Source: CAD feature listing. Evaluate the final solid. Frame: model axes, mm. A direction names the side the tool comes from. Give positions to 0.01 mm unless a question says otherwise; leave off trailing zeros. Order: outer loops, then holes, each group sorted by start corner. A loop starts at its lowest first (then second) coordinate and runs counter-clockwise, first axis right, second up.
from build123d import *

# Parameters (mm, degrees)
SKETCH1_W           = 500
SKETCH1_H           = 150
BOSS_EXTRUDE1_DEPTH = 10
SKETCH2_R           = 25.831615562
CUT_EXTRUDE1_DEPTH  = 10
SKETCH3_W           = 401.190926376
SKETCH3_H           = 128.182737921
CUT_EXTRUDE2_DEPTH  = 10
SKETCH5_W           = 641.31413219
SKETCH5_H           = 43.634524158
CUT_EXTRUDE3_DEPTH  = 10


with BuildPart() as part:
    # Sketch1 → Boss-Extrude1 (new body)
    with BuildSketch(Plane.XY):
        Rectangle(SKETCH1_W, SKETCH1_H)
    extrude(amount=BOSS_EXTRUDE1_DEPTH)

    # Sketch2 → Cut-Extrude1 (cut)
    with BuildSketch(Plane.XY.offset(10)):
        with Locations((195.256623511, 25)):
            Circle(SKETCH2_R)
    extrude(amount=-CUT_EXTRUDE1_DEPTH, mode=Mode.SUBTRACT)

    # Sketch3 → Cut-Extrude2 (cut)
    with BuildSketch(Plane.XY.offset(10)):
        with Locations((-49.404536812, 10.908631039)):
            Rectangle(SKETCH3_W, SKETCH3_H)
    extrude(amount=-CUT_EXTRUDE2_DEPTH, mode=Mode.SUBTRACT)

    # Sketch5 → Cut-Extrude3 (cut)
    with BuildSketch(Plane.XY.offset(10)):
        with Locations((-250, -53.182737921)):
            Rectangle(SKETCH5_W, SKETCH5_H)
    extrude(amount=-CUT_EXTRUDE3_DEPTH, mode=Mode.SUBTRACT)


solid = part.part
(1) Access query for faces 4 (the flat face through (110, -53.183, 5)), 5 (the flat face through (70.657, -64, 5)). Directions: +Z, -Z, +X, -X, +Y, -Y. A direction counts if a zero-diameter tool reaches every point of the face in a straight line with its end or side. Return the directions, or none.
(2) Section D-D, the plane y = -26. Return loops of the section in (x, z), plus the area to 3 significant figures.
(3) Section B-B, the plane z = 4. Return loops of the section in (x, y).
(4) Line query: line 1 along X through (y, z) = (-27, 3.75); line 2 along Y through (x, z) = (104, 5.75); line 3 along Y through (x, z) = (178.5, 1). Output: solid intervals per line, ascending.
(5) Section C-C, the plane x = 186.5. Return loops of the section in (y, z).
(6) Section A-A, the plane y = 25. Return loops of the section in (x, z) (3 decimals).
(7) Draft query along X for faces 1 (the cylindrical face through (174.76, 9.28, 5.07)), 2 (the flat face through (250, -1, 5)), 3 (the flat face through (200, 75, 5)). Return one class per face: +X half, -X half, draft (parallel to the pull), parting line (faces both ways), or undercut.
(8) Pin query (flat end, axial travel): pin 1 Ø1.5 at (y, z) = (18, 8) entering from -X. Return the tip coordinate at first contact, or that it passes through.
Checks:
1. face 4: +Z, -Z, -X, +Y
1. face 5: +Z, -Z, -X, +Y, -Y
2. outline: (151.19, 0) - (250, 0) - (250, 10) - (151.19, 10) - close
2. area: 988 mm2
3. outline: (70.66, -75) - (250, -75) - (250, 75) - (151.19, 75) - (151.19, -53.18) - (70.66, -53.18) - close; hole circle Ø51.66 at (195.26, 25)
4. line 1: x = 151.19 to 250
4. line 2: y = -75 to -53.18
4. line 3: y = -75 to 5.34, 44.66 to 75
5. outline: (-75, 0) - (0.7, 0) - (0.7, 10) - (-75, 10) - close; (49.3, 0) - (75, 0) - (75, 10) - (49.3, 10) - close
6. outline: (151.191, 0) - (169.425, 0) - (169.425, 10) - (151.191, 10) - close; (221.088, 0) - (250, 0) - (250, 10) - (221.088, 10) - close
7. face 1: undercut
7. face 2: +X half
7. face 3: draft
8. pin 1: stops at x = 151.19
